```python
from build123d import *

# Parameters (mm, degrees)
F1_FACE_R = 12.7
F2_DEPTH  = 25.4
F3_R      = 11.43
F4_DEPTH  = 25.4


with BuildPart() as f1:
    # F0 (on Front) → F1 (revolve)
    with BuildSketch(Plane.XZ):
        Polygon((0, -9.356778), (12.7, -9.356778), (12.7, 16.043222), (66.294158, 70.210613), (64.797749, 71.691186), (63.332844, 70.210613), (9.738686, 16.043222), (0, 16.043222), align=None)
    revolve(axis=Axis((0, 0, 3.343222), (0, 0, 1)))

    # F1_face (on face) → F2 (cut)
    with BuildSketch(Plane(origin=(0, 0, -9.356778), x_dir=(1, 0, 0), z_dir=(0, 0, -1))):
        Circle(F1_FACE_R)
    extrude(amount=F2_DEPTH, mode=Mode.SUBTRACT)

    # F3 (on face) → F4 (cut)
    with BuildSketch(Plane(origin=(0, 0, -9.356778), x_dir=(1, 0, 0), z_dir=(0, 0, -1))):
        Circle(F3_R)
    extrude(amount=-F4_DEPTH, mode=Mode.SUBTRACT)


solid = f1.part
```
Geometry check sheet. Reference: the model listing, model coordinates, mm. Round coordinates to 2 decimals unless told otherwise and drop trailing zeros. Loops run counter-clockwise (first coordinate to the right, second up) from the corner with the lowest first, then second, coordinate; pieces in that order, holes last. Notation, with made-up numbers: (-25, 82) - (32, 82) arc R25 ccw to (32, 105) - close; hole circle Ø6 at (30, 80). An arc over 180 degrees is marked (long way). Write item = value, one per line. Start each with the question number.
1. Section check A-A on x = 0. Enter the section's corners in (y, z).
2. Thickness scan on line 1 (Y direction, x = 0, z = 8.75); line 2 (X direction, y = 8, z = 62.5); line 3 (Y direction, x = -5.5, z = 11). Record the ranges inside material, lowest first.
3. Section check C-C on z = 63. Enter the section's corners in (x, y), then the cut area to 3 significant figures.
4. Section check D-D on z = 51.5. Enter the section's corners in (x, y), then the cut area to 3 significant figures.
5. Depth check by flat-ended pin: pin 1 (1.5 mm diameter, centred on y = -15.5, z = 60.5, fed in from -X); pin 2 (6 mm diameter, centred on y = 40, z = 50, fed in from -X); pin 3 (6 mm diameter, centred on x = -19, y = 30.5, fed in from -Z); pin 4 (13.5 mm diameter, centred on x = 0, y = 0, fed in from +Z). Enter the tip coordinate at first touch or a pass-through.
6. Mould release check, pull along X, two halves, no side actions. Record for faces 1 (the face through (-5, -9, 16.043)), 2 (the face through (-2.75, -12.4, 3.52)): released by +X, released by -X, zero draft, split by the parting line, or undercut.
Working result:
q1.outline = (-66.29, 70.21) - (-12.7, 16.04) - (-12.7, -9.36) - (-11.43, -9.36) - (-11.43, 16.04) - (-9.74, 16.04) - (-63.33, 70.21) - (-64.8, 71.69) - close; (9.74, 16.04) - (11.43, 16.04) - (11.43, -9.36) - (12.7, -9.36) - (12.7, 16.04) - (66.29, 70.21) - (64.8, 71.69) - (63.33, 70.21) - close
q2.line_1 = -12.7 to -11.43, 11.43 to 12.7
q2.line_2 = -58.12 to -55.13, 55.13 to 58.12
q2.line_3 = -11.45 to -10.02, 10.02 to 11.45
q3.outline = circle Ø118.32 at (0, 0); hole circle Ø112.4 at (0, 0)
q3.area = 1,070 mm^2
q4.outline = circle Ø95.56 at (0, 0); hole circle Ø89.64 at (0, 0)
q4.area = 861 mm^2
q5.pin_1 = -55.32
q5.pin_2 = -30.16
q5.pin_3 = 36.49
q5.pin_4 = through
q6.face_1 = undercut
q6.face_2 = split by the parting line
